Source: three-view drawing plus pictorial views. Frame: mm from the lowest corner of the part. A direction names the side the tool comes from. Coordinates: 2 decimals unless noted, no trailing zeros. Order: outer loops, then holes, each group sorted by start corner. A loop starts at its lowest first (then second) coordinate and runs counter-clockwise, first axis right, second up. Notation, with made-up numbers: M -32.5,-20 L -8.5,-20 A33 ccw -8.5,11 Z; hole C 28,-39 d7. An arc over 180 degrees is marked long. One line per question, with ' | ' between items.
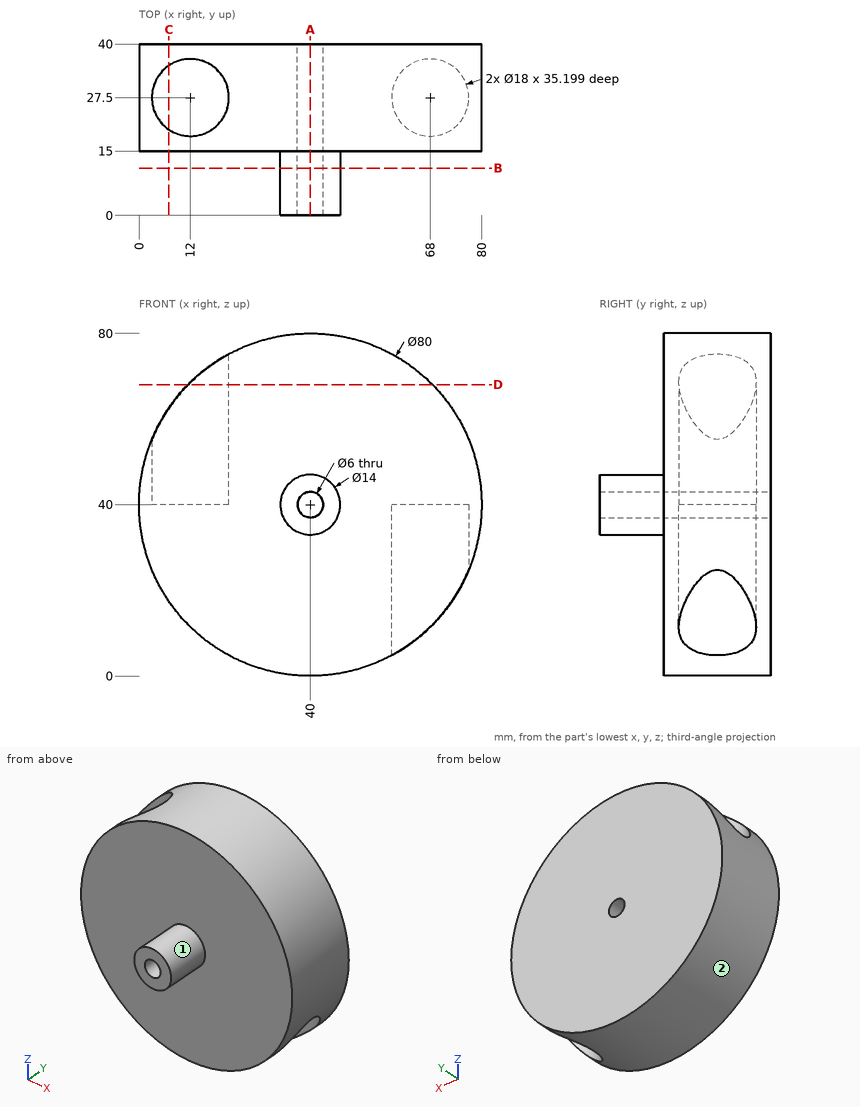
1. Section B-B, the plane y = 11. Output: boundary loops of the cut face in (x, z).
Response values:
outline: C 40,40 d14; hole C 40,40 d6
2. Pin query (flat end, axial travel): P1, Ø2, axis at x = 55.5, z = 17, coming from the -Y side; P2, Ø3, axis at y = 20, z = 14.5, coming from the +X side; P3, Ø5, axis at y = 27.5, z = 23, coming from the +X side. Return the tip coordinate at first contact, or that it passes through.
Response values:
P1: stops at y = 15 | P2: stops at x = 71.9 | P3: stops at x = 77.28
3. Section C-C, the plane x = 7. Output: boundary loops of the cut face in (y, z) (1 decimal).
Response values:
outline: M 15,17.4 L 40,17.4 L 40,62.6 L 35,62.6 L 35,40 L 20,40 L 20,62.6 L 15,62.6 Z
4. Section D-D, the plane z = 68. Output: boundary loops of the cut face in (x, y) (1 decimal), and give its area (3 significant figures).
Response values:
outline: M 11.4,15 L 68.6,15 L 68.6,40 L 11.4,40 L 11.4,36.5 A9 cw long 11.4,18.5 Z | area: 1,290 mm^2
5. Material intervals for line 1 (Z direction, x = 40, y = 11); line 2 (Z direction, x = 40, y = 25.5); line 3 (Y direction, x = 12, z = 55), sorted ascending. Write a range as [from, to].
Response values:
line 1: z = [33, 37], [43, 47] | line 2: z = [0, 37], [43, 80] | line 3: y = [15, 18.5], [36.5, 40]
6. Access query for the marked faces 1 and 2. Directions: +Z, -Z, +X, -X, +Y, -Y. A direction counts if a zero-diameter tool reaches every point of the face in a straight line with its end or side. Return the directions, or none.
Response values:
face 1: -Y | face 2: +Y, -Y
7. Section A-A, the plane x = 40. Output: boundary loops of the cut face in (y, z), and give its area (3 significant figures).
Response values:
outline: M 0,33 L 15,33 L 15,0 L 40,0 L 40,37 L 0,37 Z; M 0,43 L 40,43 L 40,80 L 15,80 L 15,47 L 0,47 Z | area: 1,970 mm^2
